Verification items for the finished model (mm, model axes). A direction names the side the tool comes from. Round coordinates to 2 decimals unless told otherwise and drop trailing zeros. Write each loop counter-clockwise with the first axis right and the second up, starting at its lowest first coordinate (ties: lowest second). Pieces come first, ordered by that corner, then holes. Notation, with made-up numbers: M 31,57 L 89,57 A17 cw 89,67 Z; hole C -15.5,0 d5. An arc over 180 degrees is marked long. One line per question, with ' | ' between items. Start each with the question number.
Q1. Cross-section at A-A (x = 34.5). Record the boundary of the cut face in (y, z).
Q2. Tool access check on faces 5 (the face through (59, 0, -20)), 6 (the face through (41, 0, -22.3)), 7 (the face through (-20, 0, -51)), 8 (the face through (20, 0, 52)). Record the directions out of +Z, -Z, +X, -X, +Y, -Y that give a thin tool (end or side, any length) a straight path to the whole face; none if there is none.
Q3. Release check for a two-part mould opening along X. For faces 1 (the face through (-39, 0, -50)), 2 (the face through (30.4, 0, -8)), 3 (the face through (20, 0, -52)), 4 (the face through (44.4, 0, 8)) record: released by +X, released by -X, zero draft, split by the parting line, or undercut.
Q4. Cross-section at B-B (x = 59). Record the boundary of the cut face in (y, z).
Q5. Cross-section at C-C (z = -51.5). Record the boundary of the cut face in (x, y), then the cut area to 3 significant figures.
Q6. Cross-section at D-D (y = 0.1). State how many separate pieces and enclosed holes the cut face has, then the cut area to 3 significant figures.
Q7. Thickness scan on line 1 along X through (y, z) = (0.25, 0); line 2 along Z through (x, y) = (36, -0.7); line 3 along X through (y, z) = (0.1, -51.5). Record the ranges inside material, lowest first. Write a range as from..to.
Q8. Gauge pin test, flat ends, axial feed: pin 1 (0.9 mm diameter, centred on x = 40.5, y = -0.5, fed in from +Z); pin 2 (1.5 mm diameter, centred on y = 0, z = 29, fed in from -X); pin 3 (1.5 mm diameter, centred on y = 0.5, z = -14.5, fed in from -X). Record the tip position at first contact, or that the pin passes through.
from build123d import *

# Parameters (mm, degrees)
ESBO_O1_W                = 115
ESBO_O1_H                = 100
RESSALTO_EXTRUS_O1_DEPTH = 1.5
RESSALTO_EXTRUS_O2_DEPTH = 3
ESBO_O2_R                = 1.5
CORTE_EXTRUS_O1_DEPTH    = 85.718652019
CUT_EXTRUDE3_DEPTH       = 85.678804904
CUT_EXTRUDE3_DEPTH_BACK  = 85.678804904
SKETCH2_W                = 16.6
SKETCH2_H                = 3


with BuildPart() as part:
    # Esboço1 → Ressalto-extrusão1 (new, symmetric)
    with BuildSketch(Plane(origin=(0, 0, 0), x_dir=(1, 0, 0), z_dir=(0, 1, 0))):
        Rectangle(ESBO_O1_W, ESBO_O1_H)
    extrude(amount=RESSALTO_EXTRUS_O1_DEPTH, both=True)

    # Esboço4 → Ressalto-extrusão2 (add, through all)
    with BuildSketch(Plane(origin=(0, 1.5, 0), x_dir=(1, 0, 0), z_dir=(0, 1, 0))):
        with BuildLine():
            Line((6.5, 53), (20, 53))
            Line((20, 53), (20, 50))
            Line((20, 50), (-20, 50))
            Line((-20, 50), (-20, 53))
            Line((-20, 53), (-6.5, 53))
            ThreePointArc((-6.5, 53), (-5.085786438, 53.585786438), (-4.5, 55))
            Line((-4.5, 55), (-4.5, 55.2))
            ThreePointArc((-4.5, 55.2), (-4.265685425, 55.765685425), (-3.7, 56))
            Line((-3.7, 56), (3.7, 56))
            ThreePointArc((3.7, 56), (4.265685425, 55.765685425), (4.5, 55.2))
            Line((4.5, 55.2), (4.5, 55))
            ThreePointArc((4.5, 55), (5.085786438, 53.585786438), (6.5, 53))
        make_face()
        with BuildLine():
            Line((-63.5, 3.7), (-63.5, -3.7))
            ThreePointArc((-63.5, -3.7), (-63.265685425, -4.265685425), (-62.7, -4.5))
            Line((-62.7, -4.5), (-62.5, -4.5))
            ThreePointArc((-62.5, -4.5), (-61.085786438, -5.085786438), (-60.5, -6.5))
            Line((-60.5, -6.5), (-60.5, -20))
            Line((-60.5, -20), (-57.5, -20))
            Line((-57.5, -20), (-57.5, 20))
            Line((-57.5, 20), (-60.5, 20))
            Line((-60.5, 20), (-60.5, 6.5))
            ThreePointArc((-60.5, 6.5), (-61.085786438, 5.085786438), (-62.5, 4.5))
            Line((-62.5, 4.5), (-62.7, 4.5))
            ThreePointArc((-62.7, 4.5), (-63.265685425, 4.265685425), (-63.5, 3.7))
        make_face()
        with BuildLine():
            Line((4.5, -55.2), (4.5, -55))
            ThreePointArc((4.5, -55), (5.085786438, -53.585786438), (6.5, -53))
            Line((6.5, -53), (20, -53))
            Line((20, -53), (20, -50))
            Line((20, -50), (-20, -50))
            Line((-20, -50), (-20, -53))
            Line((-20, -53), (-6.5, -53))
            ThreePointArc((-6.5, -53), (-5.085786438, -53.585786438), (-4.5, -55))
            Line((-4.5, -55), (-4.5, -55.2))
            ThreePointArc((-4.5, -55.2), (-4.265685425, -55.765685425), (-3.7, -56))
            Line((-3.7, -56), (3.7, -56))
            ThreePointArc((3.7, -56), (4.265685425, -55.765685425), (4.5, -55.2))
        make_face()
        with BuildLine():
            Line((57.5, 20), (60.5, 20))
            Line((60.5, 20), (60.5, 6.5))
            ThreePointArc((60.5, 6.5), (61.085786438, 5.085786438), (62.5, 4.5))
            Line((62.5, 4.5), (62.7, 4.5))
            ThreePointArc((62.7, 4.5), (63.265685425, 4.265685425), (63.5, 3.7))
            Line((63.5, 3.7), (63.5, -3.7))
            ThreePointArc((63.5, -3.7), (63.265685425, -4.265685425), (62.7, -4.5))
            Line((62.7, -4.5), (62.5, -4.5))
            ThreePointArc((62.5, -4.5), (61.085786438, -5.085786438), (60.5, -6.5))
            Line((60.5, -6.5), (60.5, -20))
            Line((60.5, -20), (57.5, -20))
            Line((57.5, -20), (57.5, 20))
        make_face()
    extrude(amount=-RESSALTO_EXTRUS_O2_DEPTH)

    # Esboço2 → Corte-extrusão1 (cut, through all)
    with BuildSketch(Plane(origin=(0, 1.5, 0), x_dir=(1, 0, 0), z_dir=(0, 1, 0))):
        with Locations(Location((0, -51.5, 0), (0, 0, 270))):
            Circle(ESBO_O2_R)
        with Locations(Location((0, 51.5, 0), (0, 0, 90))):
            Circle(ESBO_O2_R)
        with Locations(Location((59, 0, 0), (0, 0, 90))):
            Circle(ESBO_O2_R)
        with Locations(Location((-59, 0, 0), (0, 0, 270))):
            Circle(ESBO_O2_R)
    extrude(amount=-CORTE_EXTRUS_O1_DEPTH, mode=Mode.SUBTRACT)

    # Sketch2 → Cut-Extrude3 (cut, two sides: drawn at the far end of the back side and taken through both)
    with BuildSketch(Plane(origin=(0, 0, 0), x_dir=(1, 0, 0), z_dir=(0, 1, 0)).offset(-CUT_EXTRUDE3_DEPTH_BACK)):
        with BuildLine():
            Line((24.7, 4.5), (29.4, 4.5))
            ThreePointArc((29.4, 4.5), (30.107106781, 4.792893219), (30.4, 5.5))
            Line((30.4, 5.5), (30.4, 11))
            ThreePointArc((30.4, 11), (30.692893219, 11.707106781), (31.4, 12))
            Line((31.4, 12), (43.4, 12))
            ThreePointArc((43.4, 12), (44.107106781, 11.707106781), (44.4, 11))
            Line((44.4, 11), (44.4, 5.5))
            ThreePointArc((44.4, 5.5), (44.692893219, 4.792893219), (45.4, 4.5))
            Line((45.4, 4.5), (54.1, 4.5))
            ThreePointArc((54.1, 4.5), (54.807106781, 4.207106781), (55.1, 3.5))
            Line((55.1, 3.5), (55.1, -3.5))
            ThreePointArc((55.1, -3.5), (54.807106781, -4.207106781), (54.1, -4.5))
            Line((54.1, -4.5), (45.4, -4.5))
            ThreePointArc((45.4, -4.5), (44.692893219, -4.792893219), (44.4, -5.5))
            Line((44.4, -5.5), (44.4, -11))
            ThreePointArc((44.4, -11), (44.107106781, -11.707106781), (43.4, -12))
            Line((43.4, -12), (31.4, -12))
            ThreePointArc((31.4, -12), (30.692893219, -11.707106781), (30.4, -11))
            Line((30.4, -11), (30.4, -5.5))
            ThreePointArc((30.4, -5.5), (30.107106781, -4.792893219), (29.4, -4.5))
            Line((29.4, -4.5), (24.7, -4.5))
            ThreePointArc((24.7, -4.5), (23.992893219, -4.207106781), (23.7, -3.5))
            Line((23.7, -3.5), (23.7, 3.5))
            ThreePointArc((23.7, 3.5), (23.992893219, 4.207106781), (24.7, 4.5))
        make_face()
        with Locations((41.3, 23.8)):
            Rectangle(SKETCH2_W, SKETCH2_H)
    extrude(amount=CUT_EXTRUDE3_DEPTH + CUT_EXTRUDE3_DEPTH_BACK, mode=Mode.SUBTRACT)


solid = part.part
Determined:
1) outline: M -1.5,-50 L 1.5,-50 L 1.5,-25.3 L -1.5,-25.3 Z; M -1.5,-22.3 L 1.5,-22.3 L 1.5,-12 L -1.5,-12 Z; M -1.5,12 L 1.5,12 L 1.5,50 L -1.5,50 Z
2) face 5: -Z, +X, +Y, -Y | face 6: +Y, -Y | face 7: -Z, -X, +Y, -Y | face 8: +Z, +X, +Y, -Y
3) face 1: zero draft | face 2: undercut | face 3: released by +X | face 4: undercut
4) outline: M -1.5,-20 L 1.5,-20 L 1.5,-1.5 L -1.5,-1.5 Z; M -1.5,1.5 L 1.5,1.5 L 1.5,20 L -1.5,20 Z
5) outline: M -20,-1.5 L -1.5,-1.5 L -1.5,1.5 L -20,1.5 Z; M 1.5,-1.5 L 20,-1.5 L 20,1.5 L 1.5,1.5 Z | area: 111 mm²
6) separate pieces: 1 | enclosed holes: 6 | area: 11,500 mm²
7) line 1: x = -63.5..-60.5, -57.5..23.7, 55.1..57.5, 60.5..63.5 | line 2: z = -50..-25.3, -22.3..-12, 12..50 | line 3: x = -20..-1.5, 1.5..20
8) pin 1: stops at z = 50 | pin 2: stops at x = -57.5 | pin 3: stops at x = -60.5
